For this review, take the finished solid that the model builds, in its own axes (mm). Face numbers are marked on the shaded views. A direction names the side the tool comes from. Round coordinates to 2 decimals unless told otherwise and drop trailing zeros. Loops run counter-clockwise (first coordinate to the right, second up) from the corner with the lowest first, then second, coordinate; pieces in that order, holes last. Notation, with made-up numbers: M 52.25,-34.75 L 104.25,-34.75 A31 cw 104.25,0.25 Z; hole C 79,55.5 d11. An arc over 180 degrees is marked long. One line per question, with ' | ' between items. Start each with the question number.
1) We need section D-D (z = 6.35). Give the boundary of the cut face in (x, y).
2) For pin 1 Ø1.5 at (x, y) = (4, 2) entering from +Z; pin 2 Ø2 at (x, y) = (5, 0.5) entering from -Z, all flat-tipped, find the tip position at first contact; note any pin that passes through.
3) We need section C-C (y = 4.25). State how many separate pieces and enclosed holes the cut face has, and give its area (3 significant figures).
4) We need section B-B (z = 0). Give the boundary of the cut face in (x, y) (3 decimals), and give its area (3 significant figures).
5) For the marked faces 1, 2 and 3, list the 3-axis set-ups (+Z, -Z, +X, -X, +Y, -Y) from which the entire face can be reached by the end or side of a thin tool; tool diameter is ignored.
6) For probe 1 along Z at (x, y) = (0, 4.5) (3 decimals); probe 2 along X at (y, z) = (2, 6.35); probe 3 along Z at (x, y) = (-2, 0.5) (3 decimals), list the stretches that pass through material, from the lowest coordinate up. Write a range as from..to.
7) We need section A-A (x = 0). Give the boundary of the cut face in (y, z) (3 decimals).
8) Mouldability with a two-part tool opening along Z and no side actions: class the marked faces 4, 5, 6 and 7 as pulls with the +Z half, pulls with the -Z half, needs draft (parallel to the pull), parting line crosses it, or undercut.
```python
from build123d import *

# Parameters (mm, degrees)
SKETCH1_R           = 2.5796875
SKETCH1_W           = 6.35
SKETCH1_H           = 6.35
BOSS_EXTRUDE1_DEPTH = 6.35


with BuildPart() as part:
    # Sketch1 → Boss-Extrude1 (new body)
    with BuildSketch(Plane(origin=(0, 0, 0), x_dir=(1, 0, 0), z_dir=(0, 1, 0))):
        with BuildLine():
            Line((-1.190625, -10.903378281), (-1.190625, -16.281552001))
            ThreePointArc((-1.190625, -16.281552001), (-2.079347575, -18.137007052), (-4.082142857, -18.607488001))
            ThreePointArc((-4.082142857, -18.607488001), (0, 19.05), (4.082142857, -18.607488001))
            ThreePointArc((4.082142857, -18.607488001), (2.079347575, -18.137007052), (1.190625, -16.281552001))
            Line((1.190625, -16.281552001), (1.190625, -10.903378281))
            ThreePointArc((1.190625, -10.903378281), (0, -9.712753281), (-1.190625, -10.903378281))
        make_face()
        with Locations((0, 12.7)):
            Circle(SKETCH1_R, mode=Mode.SUBTRACT)
        with Locations((10.998522628, -6.35)):
            Circle(SKETCH1_R, mode=Mode.SUBTRACT)
        with Locations((-10.998522628, -6.35)):
            Circle(SKETCH1_R, mode=Mode.SUBTRACT)
        Rectangle(SKETCH1_W, SKETCH1_H, mode=Mode.SUBTRACT)
    extrude(amount=BOSS_EXTRUDE1_DEPTH)


solid = part.part
```
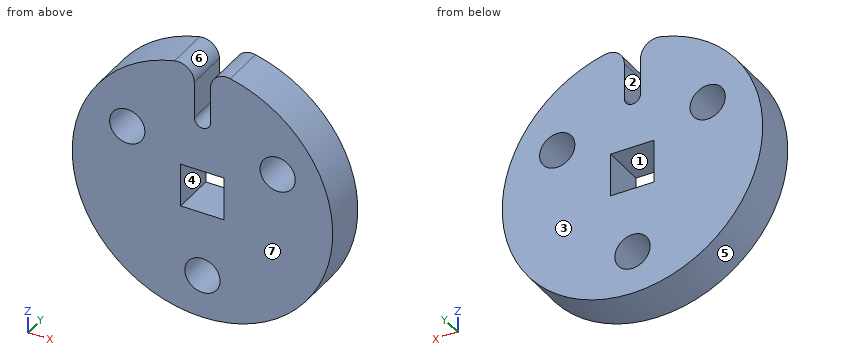
Answers below:
1) outline: M -17.96,0 L -13.58,0 L -13.58,6.35 L -17.96,6.35 Z; M -8.42,0 L 8.42,0 L 8.42,6.35 L -8.42,6.35 Z; M 13.58,0 L 17.96,0 L 17.96,6.35 L 13.58,6.35 Z
2) pin 1: z = 18.66 | pin 2: z = -18.63
3) separate pieces: 1 | enclosed holes: 4 | area: 1,010 mm^2
4) outline: M -19.05,0 L -3.175,0 L -3.175,6.35 L -19.05,6.35 Z; M 3.175,0 L 19.05,0 L 19.05,6.35 L 3.175,6.35 Z | area: 202 mm^2
5) face 1: +Y, -Y | face 2: +Z, +Y, -Y | face 3: +Z, -Z, +X, -X, +Y
6) probe 1: -19.05..-15.28, -10.12..-3.175, 3.175..9.713 | probe 2: -17.96..-13.58, -8.42..8.42, 13.58..17.96 | probe 3: -18.945..-14.329, -11.071..-3.175, 3.175..18.07
7) outline: M 0,-19.05 L 6.35,-19.05 L 6.35,-15.28 L 0,-15.28 Z; M 0,-10.12 L 6.35,-10.12 L 6.35,-3.175 L 0,-3.175 Z; M 0,3.175 L 6.35,3.175 L 6.35,9.713 L 0,9.713 Z
8) face 4: undercut | face 5: parting line crosses it | face 6: pulls with the +Z half | face 7: needs draft
